Autodesk Inventor part; units mm, degrees
ref_plane "YZ Plane" through (0, 0, 0) normal (1, 0, 0) x (0, 1, 0)
ref_plane "XZ Plane" through (0, 0, 0) normal (0, 1, 0) x (-1, 0, 0)
ref_plane "XY Plane" through (0, 0, 0) normal (0, 0, 1) x (1, 0, 0)
sketch "Эскиз1" plane through (0, 0, 0) normal (0, 0, 1) x (1, 0, 0)
  circle A0 centre (-7.5, -22.95) radius 1.5
  circle A1 centre (7.5, -22.95) radius 1.5
  circle A2 centre (7.5, -6.95) radius 1.5
  circle A3 centre (-7.5, -6.95) radius 1.5
  line L0 (-281.4, 13.05) -> (10, 13.05)
  line L1 (10, 13.05) -> (10, -42.95)
  line L2 (10, -42.95) -> (-281.4, -42.95)
  line L3 (-281.4, -42.95) -> (-281.4, 13.05)
  line L4 (-281.4, 13.05) -> (10, -42.95) construction
  line L5 (10, 13.05) -> (-281.4, -42.95) construction
  line L6 (-135.7, -14.95) -> (-135.7, -42.95) construction
  circle A4 centre (-263.9, -22.95) radius 1.5
  circle A5 centre (-278.9, -22.95) radius 1.5
  circle A6 centre (-278.9, -6.95) radius 1.5
  circle A7 centre (-263.9, -6.95) radius 1.5
  point P0 (0, 0)
  dimension "d5" = 291.4
  dimension "d8" = 2.5
  dimension "d9" = 20
  dimension "d10" = 20
extrude "Выдавливание1" add sketch "Эскиз1" along normal blind 4
sketch "Эскиз4" plane through (0, 0, 0) normal (0, 0, -1) x (-1, 0, 0)
  line L0 (27.7, 31.05) -> (243.7, 31.05)
  line L1 (243.7, 31.05) -> (243.7, -4.95)
  line L2 (243.7, -4.95) -> (27.7, -4.95)
  line L3 (27.7, -4.95) -> (27.7, 31.05)
  line L4 (-10, 13.05) -> (281.4, 13.05)
  line L5 (27.7, 31.05) -> (243.7, -4.95) construction
  line L6 (243.7, 31.05) -> (27.7, -4.95) construction
  point P0 (0, 0)
  point P1 (135.7, 13.05)
  point P2 (243.7, 13.05)
  dimension "d13" = 18
  dimension "d14" = 216
extrude "Выдавливание3" cut sketch "Эскиз4" against normal blind 4
ref_plane "РабПлоскость1" through (-281.4, -14.95, 0) normal (0, -1, 0) x (1, 0, 0)
mirror "Зеркальное отражение1" about plane through (-281.4, -14.95, 0) normal (0, -1, 0) of "Выдавливание3"
sketch "Эскиз8" plane through (0, 0, 4) normal (0, 0, 1) x (1, 0, 0)
  circle A0 centre (-278.8, -36.95) radius 1.6
  line L0 (-243.7, -42.95) -> (-243.7, -24.95)
  line L1 (-281.4, -42.95) -> (-243.7, -42.95)
  circle A1 centre (-278.8, 7.05) radius 1.6
  point P0 (0, 0)
  dimension "d48" = 3.2
  dimension "d49" = 44
extrude "Выдавливание7" cut sketch "Эскиз8" against normal blind 10
ref_plane "РабПлоскость2" through (-135.7, -42.95, 0) normal (-1, 0, 0) x (0, 0, 1)
mirror "Зеркальное отражение2" about plane through (-135.7, -42.95, 0) normal (-1, 0, 0) of "Выдавливание7"
sketch "Эскиз10" plane through (0, 0, 4) normal (0, 0, 1) x (1, 0, 0)
  circle A0 centre (7.4, -36.95) radius 1.6
  circle A1 centre (-25.1, -36.95) radius 1.6
  point P0 (0, 0)
  dimension "d50" = 3.2
  dimension "d51" = 32.5
extrude "Выдавливание8" cut sketch "Эскиз10" against normal blind 10
sketch "Эскиз11" plane through (0, 0, 4) normal (0, 0, 1) x (1, 0, 0)
  circle A0 centre (-256.6, 9.05) radius 1.6
  point P0 (0, 0)
extrude "Выдавливание9" cut sketch "Эскиз11" against normal blind 10
mirror "Зеркальное отражение4" about plane through (-135.7, -42.95, 0) normal (-1, 0, 0) of "Выдавливание9"
sketch "Эскиз12" plane through (0, 0, 4) normal (0, 0, 1) x (1, 0, 0)
  circle A0 centre (-14.8, -14.95) radius 1.6
  line L0 (-243.7, -24.95) -> (-27.7, -24.95)
  circle A1 centre (-14.8, 9.05) radius 1.6
  line L1 (-14.8, -24.95) -> (-14.8, 9.05) construction
  circle A2 centre (-60.5, -14.95) radius 1.6
  circle A3 centre (-46.3, -14.95) radius 1.6
  point P0 (0, 0)
  dimension "d56" = 3.2
  dimension "d57" = 10
  dimension "d58" = 3.2
  dimension "d59" = 45.7
extrude "Выдавливание10" cut sketch "Эскиз12" against normal blind 10 contours A0 | A2 | A3
properties part number "центр_рейка" material "Древесина (береза)"
Source: CAD feature listing. Evaluate the final solid. Frame: model axes, mm. Give positions to 0.01 mm unless a question says otherwise; leave off trailing zeros. Order: outer loops, then holes, each group sorted by start corner. A loop starts at its lowest first (then second) coordinate and runs counter-clockwise, first axis right, second up. Notation, with made-up numbers: (13.25, -20) -> (62.25, -20) arc R24 ccw to (62.25, -1) -> close; hole circle Ø2 at (17.25, 3). An arc over 180 degrees is marked (long way). Use a Markdown table: item, result.
1) Contact query for flat-ended pins moving along their axis: P1, Ø5, axis at x = -200, y = -15.5, coming from the -Z side; P2, Ø1, axis at x = -103, z = 1, coming from the -Y side. Output: stop coordinate, or through.
Answer list:
| item | result |
|---|---|
| P1 | z = 0 |
| P2 | y = -24.95 |
2) Section query C-C, the plane x = -195.5. Return the cut outline in (y, z).
Answer list:
| item | result |
|---|---|
| outline | (-24.95, 0) -> (-4.95, 0) -> (-4.95, 4) -> (-24.95, 4) -> close |
3) Ray query, line 1 along Y through (x, z) = (-278.9, 1.3); line 2 along Y through (x, z) = (-7.5, 1); line 3 along X through (y, z) = (-7, 0.8). Return the intervals inside material, ascending. Write a range as [from, to].
Answer list:
| item | result |
|---|---|
| line 1 | [-42.95, -38.55], [-35.35, -24.45], [-21.45, -8.45], [-5.45, 5.45], [8.65, 13.05] |
| line 2 | [-42.95, -24.45], [-21.45, -8.45], [-5.45, 13.05] |
| line 3 | [-281.4, -280.4], [-277.4, -265.4], [-262.4, -9], [-6, 6], [9, 10] |
4) Section query B-B, the plane z = 0.75. Count the separate pieces of the cut face and the enclosed holes in it, then the cut area to 3 significant figures.
Answer list:
| item | result |
|---|---|
| separate pieces | 1 |
| enclosed holes | 18 |
| area | 8,410 mm² |
5) Section query A-A, the plane y = 3. Return the cut outline in (x, z).
Answer list:
| item | result |
|---|---|
| outline | (-281.4, 0) -> (-243.7, 0) -> (-243.7, 4) -> (-281.4, 4) -> close; (-27.7, 0) -> (10, 0) -> (10, 4) -> (-27.7, 4) -> close |
